Can you work these out from the model? Positions are in its coordinate system, mm. Coordinates: 2 decimals unless noted, no trailing zeros. Write each loop counter-clockwise with the first axis right and the second up, starting at its lowest first coordinate (ties: lowest second). Pieces come first, ordered by that corner, then holes.
```python
from build123d import *

# Parameters (mm, degrees)
CUT_EXTRUDE1_DEPTH      = 14
CUT_EXTRUDE1_DEPTH_BACK = 14


with BuildPart() as part:
    # Sketch1 → Revolve1 (revolve)
    with BuildSketch(Plane(origin=(0, 0, 0), x_dir=(0, 0, -1), z_dir=(1, 0, 0)), mode=Mode.PRIVATE) as revolve1_sk:
        Polygon((-25.5, 0), (-25.5, 6.5), (-25, 7), (-17.5, 7), (-17.5, 9.422649731), (-16.5, 10), (386.333333333, 10), (386.333333333, 16), (397, 16), (397, 0), align=None)
    revolve(revolve1_sk.sketch.rotate(Axis((0, 0, -397), (0, 0, 1)), 270), axis=Axis((0, 0, -397), (0, 0, 1)))

    # Sketch2 → Cut-Extrude1 (cut, two sides: drawn at the far end of the back side and taken through both)
    with BuildSketch(Plane(origin=(0, 0, 0), x_dir=(1, 0, 0), z_dir=(0, 1, 0)).offset(-CUT_EXTRUDE1_DEPTH_BACK)):
        Polygon((-8, -18.5), (-8, -28.5), (8, -28.5), (8, -18.5), (5, -18.5), (5, -25.5), (-5, -25.5), (-5, -18.5), align=None)
    extrude(amount=CUT_EXTRUDE1_DEPTH + CUT_EXTRUDE1_DEPTH_BACK, mode=Mode.SUBTRACT)

    # Sketch3 → Revolve2 (revolve)
    with BuildSketch(Plane(origin=(0, 0, 0), x_dir=(0, 0, -1), z_dir=(1, 0, 0)), mode=Mode.PRIVATE) as revolve2_sk:
        with BuildLine():
            Line((-47.5, 0), (-47.5, 4.233))
            Line((-47.5, 4.233), (-46.733, 5))
            Line((-46.733, 5), (-29.267, 5))
            Line((-29.267, 5), (-28.5, 4.233))
            Line((-28.5, 4.233), (-26.1, 4.233))
            ThreePointArc((-26.1, 4.233), (-25.675735931, 4.408735931), (-25.5, 4.833))
            Line((-25.5, 4.833), (-25.5, 0))
            Line((-25.5, 0), (-47.5, 0))
        make_face()
    revolve(revolve2_sk.sketch.rotate(Axis((0, 0, 25.5), (0, 0, 1)), 270), axis=Axis((0, 0, 25.5), (0, 0, 1)))


solid = part.part
```
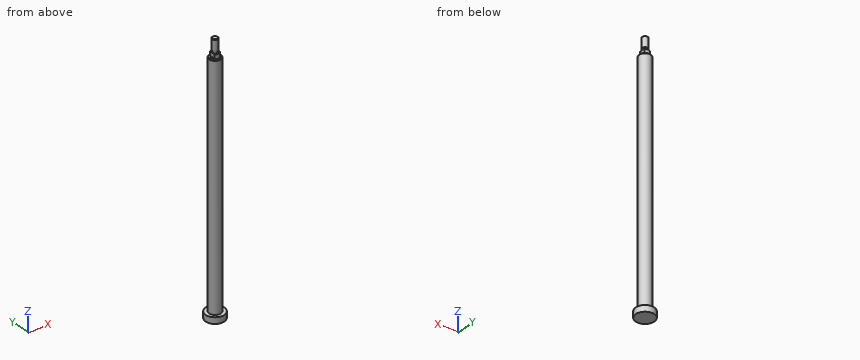
1. If we section it at C-C, the plane z = -229: List the corners of the cut face in (x, y) for me, plus the area to 3 significant figures.
2. If we section it at A-A, the plane x = 0: List the corners of the cut face in (y, z) for me, plus the area to 3 significant figures.
3. If I drill on L1, parallel to Z at x = 9, y = 0; L2, parallel to Z at x = -10, y = -5; L3, parallel to Y at x = -0.5, z = 15, over which ranges is the centre line in solid material (lowest first)?
4. I'm going to push flat-ended pins straight in: P1, Ø4, axis at y = 7, z = -18, coming from the +X side; P2, Ø1, axis at x = 6, y = -0.5, coming from the +Z side; P3, Ø8, axis at y = 12.5, z = -177.5, coming from the +X side. Where does each tip first touch, or does it pass through?
Answers:
1. outline: circle Ø20 at (0, 0)
1. area: 314 mm2
2. outline: (-16, -397) - (16, -397) - (16, -386.33) - (10, -386.33) - (10, 16.5) - (9.42, 17.5) - (7, 17.5) - (7, 25) - (6.5, 25.5) - (4.83, 25.5) arc R0.6 cw to (4.23, 26.1) - (4.23, 28.5) - (5, 29.27) - (5, 46.73) - (4.23, 47.5) - (-4.23, 47.5) - (-5, 46.73) - (-5, 29.27) - (-4.23, 28.5) - (-4.23, 26.1) arc R0.6 cw to (-4.83, 25.5) - (-6.5, 25.5) - (-7, 25) - (-7, 17.5) - (-9.42, 17.5) - (-10, 16.5) - (-10, -386.33) - (-16, -386.33) - close
2. area: 8,740 mm2
3. L1: z = -397 to 17.5
3. L2: z = -397 to -386.33
3. L3: y = -9.99 to 9.99
4. P1: stops at x = 8.66
4. P2: stops at z = 18.5
4. P3: stops at x = 5.27
